Verification items for the finished model (mm, model axes). Face numbers are marked on the shaded views. A direction names the side the tool comes from. Round coordinates to 2 decimals unless told otherwise and drop trailing zeros. Order: outer loops, then holes, each group sorted by start corner. A loop starts at its lowest first (then second) coordinate and runs counter-clockwise, first axis right, second up. Notation, with made-up numbers: (52, -29) -> (88, -29) arc R21 ccw to (88, -8) -> close; hole circle Ø3 at (4.5, -37). An arc over 180 degrees is marked (long way). Return JSON: item names as keys, results as strings. Group by question number.
Item 1: Sectioned sample at C-C on x = 65. Record the cut outline in (y, z), plus the area to 3 significant figures.
Item 2: Depth check by flat-ended pin: pin 1 Ø6 at (y, z) = (-2.5, -1.5) entering from -X; pin 2 Ø10 at (x, y) = (51, 13) entering from -Z; pin 3 Ø10 at (x, z) = (16, -13) entering from +Y; pin 4 Ø8 at (y, z) = (6.5, 11) entering from +X. Enter the tip coordinate at first touch or a pass-through.
Item 3: Scan lines: probe 1 along X at (y, z) = (14, 6.5); probe 2 along Z at (x, y) = (23, -8); probe 3 along X at (y, z) = (18, -0.5). Record each from-to range of solid material in increasing order. Write a range as from..to.
Item 4: Draft check along Z on the marked faces 5, 6 and 7. Enter one of: pulls with the +Z half, pulls with the -Z half, needs draft (parallel to the pull), parting line crosses it, or undercut.
Item 5: Access from +Z, -Z, +X, -X, +Y, -Y to the whole of each face (thin tool, end or side, straight path). Record for the marked faces 1, 2, 3 and 4.
Item 6: Sectioned sample at A-A on x = 18.5. Record the cut outline in (y, z), plus the area to 3 significant figures.
Item 7: Sectioned sample at B-B on x = 40. Record the cut outline in (y, z).
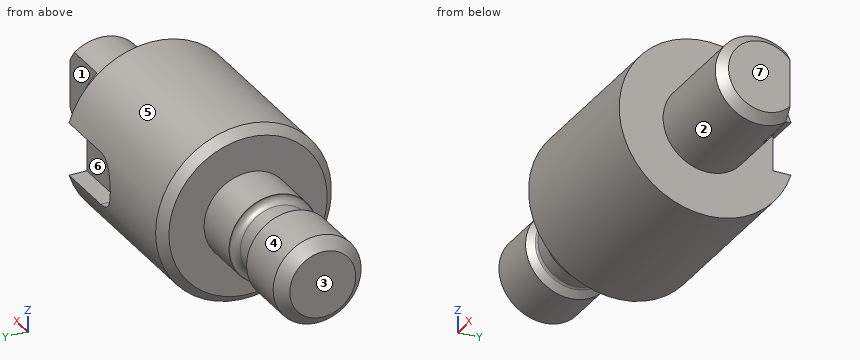
Autodesk Inventor part; units mm, degrees
ref_plane "YZ Plane" through (0, 0, 0) normal (1, 0, 0) x (0, 1, 0)
ref_plane "XZ Plane" through (0, 0, 0) normal (0, 1, 0) x (-1, 0, 0)
ref_plane "XY Plane" through (0, 0, 0) normal (0, 0, 1) x (1, 0, 0)
sketch "Эскиз1" plane through (0, 0, 0) normal (0, 0, 1) x (1, 0, 0)
  line L0 (-20, 0) -> (120, 0)
  line L1 (0, -4) -> (0, 24)
  line L2 (0, 0) -> (0, 10)
  line L3 (0, 10) -> (16, 10)
  line L4 (16, 10) -> (16, 8.25)
  line L5 (16, 8.25) -> (22, 8.25)
  line L6 (22, 8.25) -> (22, 10)
  line L7 (22, 10) -> (33, 10)
  line L8 (33, 10) -> (33, 20)
  line L9 (33, 20) -> (75, 20)
  line L10 (75, 20) -> (75, 10)
  line L11 (75, 10) -> (100, 10)
  line L12 (100, 10) -> (100, 0)
  line L13 (100, 0) -> (0, 0)
  dimension "d0" = 20
  dimension "d1" = 16.5
  dimension "d2" = 20
  dimension "d3" = 6
  dimension "d4" = 22
  dimension "d5" = 100
  dimension "d6" = 25
  dimension "d7" = 42
  dimension "d8" = 40
  dimension "d9" = 20
revolve "Вращение1" add sketch "Эскиз1" angle 360 about axis through (-10, 0, 0) along (1, 0, 0)
thread "Резьба1"
chamfer "Фаска1" distance 2.5 angle 45 1 edges at (0, -10, 0)
sketch "Эскиз2" plane through (0, 0, 0) normal (0, 0, 1) x (1, 0, 0)
  line L0 (0, 7.5) -> (2.5, 10)
  line L1 (2.5, 10) -> (16, 10)
  line L2 (16, 10) -> (16, 8.25)
  line L3 (16, 8.25) -> (22, 8.25)
  line L4 (22, 8.25) -> (22, 10)
  line L5 (22, 10) -> (33, 10)
  line L6 (33, 10) -> (33, 20)
  line L7 (33, 20) -> (75, 20)
  line L8 (75, 20) -> (75, 10)
  line L9 (75, 10) -> (100, 10)
  line L10 (100, 10) -> (100, -10)
  line L11 (100, -10) -> (75, -10)
  line L12 (75, -10) -> (75, -20)
  line L13 (75, -20) -> (33, -20)
  line L14 (33, -20) -> (33, -10)
  line L15 (33, -10) -> (22, -10)
  line L16 (22, -10) -> (22, -8.25)
  line L17 (22, -8.25) -> (16, -8.25)
  line L18 (16, -8.25) -> (16, -10)
  line L19 (16, -10) -> (2.5, -10)
  line L20 (2.5, -10) -> (0, -7.5)
  line L21 (0, -7.5) -> (0, 7.5)
  line L22 (16, 8.25) -> (14.25, 10)
  line L23 (16, 10) -> (14.25, 10)
  line L24 (16, 10) -> (16, 8.25)
  line L25 (-20, 0) -> (120, 0)
  point P0 (0, 0)
revolve "Вращение2" cut sketch "Эскиз2" angle 360 about axis through (-10, 0, 0) along (1, 0, 0) contours L1 L2 L22
fillet "Сопряжение1" radius 1 1 edges at (16, -8.25, 0)
fillet "Сопряжение2" radius 1.6 1 edges at (22, -8.25, 0)
chamfer "Фаска2" distance 2 angle 45 1 edges at (33, -20, 0)
chamfer "Фаска3" distance 2 angle 45 1 edges at (100, -10, 0)
sketch "Эскиз3" plane through (0, 0, 0) normal (0, 0, 1) x (1, 0, 0)
  line L0 (0, 7.5) -> (2.5, 10)
  line L1 (2.5, 10) -> (14.25, 10)
  line L2 (14.25, 10) -> (15.7071, 8.5429)
  arc A0 (15.7071, 8.5429) -> (16.4142, 8.25) centre (16.4142, 9.25) ccw
  line L3 (16.4142, 8.25) -> (20.4, 8.25)
  arc A1 (20.4, 8.25) -> (22, 9.85) centre (20.4, 9.85) ccw
  line L4 (22, 9.85) -> (22, 10)
  line L5 (22, 10) -> (33, 10)
  line L6 (33, 10) -> (33, 18)
  line L7 (33, 18) -> (35, 20)
  line L8 (35, 20) -> (75, 20)
  line L9 (75, 20) -> (75, 10)
  line L10 (75, 10) -> (98, 10)
  line L11 (98, 10) -> (100, 8)
  line L12 (100, 8) -> (100, -8)
  line L13 (100, -8) -> (98, -10)
  line L14 (98, -10) -> (75, -10)
  line L15 (75, -10) -> (75, -20)
  line L16 (75, -20) -> (35, -20)
  line L17 (35, -20) -> (33, -18)
  line L18 (33, -18) -> (33, -10)
  line L19 (33, -10) -> (22, -10)
  line L20 (22, -10) -> (22, -9.85)
  arc A2 (22, -9.85) -> (20.4, -8.25) centre (20.4, -9.85) ccw
  line L21 (20.4, -8.25) -> (16.4142, -8.25)
  arc A3 (16.4142, -8.25) -> (15.7071, -8.5429) centre (16.4142, -9.25) ccw
  line L22 (15.7071, -8.5429) -> (14.25, -10)
  line L23 (14.25, -10) -> (2.5, -10)
  line L24 (2.5, -10) -> (0, -7.5)
  line L25 (0, -7.5) -> (0, 7.5)
  line L26 (100, 6) -> (88, 6)
  line L27 (88, 6) -> (88, 10)
  line L28 (88, 10) -> (88, 15)
  line L29 (88, 15) -> (103, 15)
  line L30 (103, 15) -> (100, 6)
  point P0 (0, 0)
  dimension "d25" = 12
  dimension "d26" = 16
  dimension "d27" = 5
  dimension "d28" = 15
extrude "Выдавливание1" cut sketch "Эскиз3" along normal mid plane 100 contours L28 L29 L30 L12 L11 L10 | L10 L11 L12 L26 L27
sketch "Эскиз4" plane through (75, 0, 0) normal (1, 0, 0) x (0, 0, -1)
  line L0 (-6, 15) -> (6, 15)
  line L1 (0, -28) -> (0, 28)
  line L2 (-6, 15) -> (-6, 25)
  line L3 (-6, 25) -> (6, 25)
  line L4 (6, 25) -> (6, 15)
  circle A0 centre (0, 0) radius 10
  circle A1 centre (0, 0) radius 20
  line L5 (0, 20) -> (6, 20) construction
  dimension "d31" = 10
  dimension "d32" = 12
  dimension "d33" = 5
extrude "Выдавливание2" cut sketch "Эскиз4" against normal blind 14 contours L2 A1 L1 L0 | L1 A1 L4 L0 | L2 L3 L1 A1 | L1 L3 L4 A1
sketch "Эскиз5" plane through (75, 15, 6) normal (0, 1, 0) x (1, 0, 0)
  line L0 (-14, 12) -> (-14, 0)
  circle A0 centre (-14, 6) radius 6
  point P0 (-75, 6)
extrude "Выдавливание3" cut sketch "Эскиз5" along normal blind 15
properties part number "Вал"
Recorded:
{
 "1": {"outline": "(15, -6) -> (15, 6) -> (19.08, 6) arc R20 ccw (long way) to (19.08, -6) -> close", "area": "1,200 mm²"},
 "2": {"pin 1": "x = 0", "pin 2": "z = -18.33", "pin 3": "y = 5.55", "pin 4": "x = 99.22"},
 "3": {"probe 1": "33..75", "probe 2": "-6..6", "probe 3": "33.01..55.02"},
 "4": {"face 5": "parting line crosses it", "face 6": "undercut", "face 7": "needs draft"},
 "5": {"face 1": "+Z, -Z, +X, +Y", "face 2": "+X", "face 3": "+Z, -Z, -X, +Y, -Y", "face 4": "-X"},
 "6": {"outline": "circle Ø16.5 at (0, 0)", "area": "214 mm²"},
 "7": {"outline": "circle Ø40 at (0, 0)"}
}
